```python
from build123d import *

# Parameters (mm, degrees)
SKETCH1_R            = 2.6
BASE_FLANGE1_DEPTH   = 1.524
KEYING_DEPTH         = 10
FILLET1_R            = 2
FILLET2_R            = 4
JOG1_START           = -33.370112718
JOG1_DEPTH           = 8.3
JOG1_2_DEPTH         = 8.3
JOG1_START_2         = 10.476
JOG1_3_DEPTH         = 1.524
CUT_EXTRUDE1_DEPTH   = 12
CUT_EXTRUDE1_START   = -1.524
CUT_EXTRUDE1_2_DEPTH = 1.524
CUT_EXTRUDE1_3_DEPTH = 1.524


with BuildPart() as part:
    # Base-Flange1: sheet metal written as solids
    # Sketch1 → Base-Flange1 (new body)
    with BuildSketch(Plane(origin=(0, 0, 0), x_dir=(0, 0, -1), z_dir=(1, 0, 0))):
        with BuildLine():
            Line((33.370112718, 22.8), (33.370112718, 64.8))
            Line((33.370112718, 64.8), (25.070112718, 64.8))
            Line((25.070112718, 64.8), (25.070112718, 21.281826676))
            Line((25.070112718, 21.281826676), (3.832112718, 9.020061659))
            Line((3.832112718, 9.020061659), (8.220112718, 1.419822715))
            Line((8.220112718, 1.419822715), (8.982112718, 0.1))
            Line((8.982112718, 0.1), (25.905336052, 9.870627547))
            ThreePointArc((25.905336052, 9.870627547), (31.369931839, 15.335223334), (33.370112718, 22.8))
        make_face()
        with Locations((29.220112718, 26.8)):
            Circle(SKETCH1_R, mode=Mode.SUBTRACT)
        with BuildLine():
            Line((31.720112718, 60.8), (31.720112718, 53.8))
            ThreePointArc((31.720112718, 53.8), (29.220112718, 51.3), (26.720112718, 53.8))
            Line((26.720112718, 53.8), (26.720112718, 60.8))
            ThreePointArc((26.720112718, 60.8), (29.220112718, 63.3), (31.720112718, 60.8))
        make_face(mode=Mode.SUBTRACT)
    extrude(amount=-BASE_FLANGE1_DEPTH)

    # Sketch6 → Keying (cut)
    with BuildSketch(Plane(origin=(0, 0, 0), x_dir=(0, 0, -1), z_dir=(1, 0, 0))):
        Polygon((19.287815023, 6.05), (17.763815023, 8.689645431), (13.953303246, 6.489645431), (10.14279147, 4.289645431), (11.66679147, 1.65), (15.701110868, 3.97921539), align=None)
    extrude(amount=-KEYING_DEPTH, mode=Mode.SUBTRACT)

    # Fillet1
    fillet1_edges = [part.edges().sort_by_distance(p)[0] for p in [
        (-0.762, 0.1, -8.982112718),
        (-0.762, 21.281826676, -25.070112718),
        (-0.762, 64.8, -25.070112718),
        (-0.762, 64.8, -33.370112718),
    ]]
    fillet(fillet1_edges, radius=FILLET1_R)

    # Fillet2
    fillet2_edges = [part.edges().sort_by_distance(p)[0] for p in [
        (-0.762, 9.020061659, -3.832112718),
    ]]
    fillet(fillet2_edges, radius=FILLET2_R)

    # Jog1: read off the stored shape, not the designer's step
    # Jog1 outline → Jog1 (cut)
    with BuildSketch(Plane.XY.offset(JOG1_START)):
        with BuildLine():
            ThreePointArc((-1.524, 33.004579798), (-1.115645431, 34.528579798), (0, 35.644225229))
            Line((0, 35.644225229), (0, 64.8))
            Line((0, 64.8), (-1.524, 64.8))
            Line((-1.524, 64.8), (-1.524, 33.004579798))
        make_face()
    extrude(amount=JOG1_DEPTH, mode=Mode.SUBTRACT)

    # Jog1 2 outline → Jog1 2 (add)
    with BuildSketch(Plane.XY.offset(JOG1_START)):
        with BuildLine():
            ThreePointArc((0, 33.004579798), (0.446369265, 34.082210533), (1.524, 34.528579798))
            Line((1.524, 34.528579798), (8.952, 34.528579798))
            ThreePointArc((8.952, 34.528579798), (11.107261469, 35.421318329), (12, 37.576579798))
            Line((12, 37.576579798), (12, 64.8))
            Line((12, 64.8), (10.476, 64.8))
            Line((10.476, 64.8), (10.476, 37.576579798))
            ThreePointArc((10.476, 37.576579798), (10.029630734, 36.498949063), (8.952, 36.052579798))
            Line((8.952, 36.052579798), (1.524, 36.052579798))
            ThreePointArc((1.524, 36.052579798), (0.73511955, 35.948721717), (0, 35.644225229))
            Line((0, 35.644225229), (0, 33.004579798))
        make_face()
    extrude(amount=JOG1_2_DEPTH)

    # Jog1 3 outline → Jog1 3 (cut)
    with BuildSketch(Plane.YZ.offset(JOG1_START_2)):
        with BuildLine():
            ThreePointArc((62.8, -25.070112718), (64.214213562, -25.655899156), (64.8, -27.070112718))
            Line((64.8, -27.070112718), (64.8, -25.070112718))
            Line((64.8, -25.070112718), (62.8, -25.070112718))
        make_face()
        with BuildLine():
            ThreePointArc((64.8, -31.370112718), (64.214213562, -32.78432628), (62.8, -33.370112718))
            Line((62.8, -33.370112718), (64.8, -33.370112718))
            Line((64.8, -33.370112718), (64.8, -31.370112718))
        make_face()
        with BuildLine():
            Line((60.8, -26.720112718), (53.8, -26.720112718))
            ThreePointArc((53.8, -26.720112718), (51.3, -29.220112718), (53.8, -31.720112718))
            Line((53.8, -31.720112718), (60.8, -31.720112718))
            ThreePointArc((60.8, -31.720112718), (63.3, -29.220112718), (60.8, -26.720112718))
        make_face()
    extrude(amount=JOG1_3_DEPTH, mode=Mode.SUBTRACT)

    # Cut-Extrude1: read off the stored shape, not the designer's step
    # Cut-Extrude1 outline → Cut-Extrude1 (cut)
    with BuildSketch(Plane(origin=(0, 0, 0), x_dir=(0, 0, -1), z_dir=(1, 0, 0))):
        with BuildLine():
            Line((25.070112718, 32), (33.370112718, 32))
            Line((33.370112718, 32), (33.370112718, 62.8))
            ThreePointArc((33.370112718, 62.8), (32.78432628, 64.214213562), (31.370112718, 64.8))
            Line((31.370112718, 64.8), (27.070112718, 64.8))
            ThreePointArc((27.070112718, 64.8), (25.655899156, 64.214213562), (25.070112718, 62.8))
            Line((25.070112718, 62.8), (25.070112718, 32))
        make_face()
        with BuildLine():
            ThreePointArc((26.720112718, 60.8), (29.220112718, 63.3), (31.720112718, 60.8))
            Line((31.720112718, 60.8), (31.720112718, 53.8))
            ThreePointArc((31.720112718, 53.8), (29.220112718, 51.3), (26.720112718, 53.8))
            Line((26.720112718, 53.8), (26.720112718, 60.8))
        make_face(mode=Mode.SUBTRACT)
    extrude(amount=CUT_EXTRUDE1_DEPTH, mode=Mode.SUBTRACT)

    # Cut-Extrude1 2 outline → Cut-Extrude1 2 (cut)
    with BuildSketch(Plane(origin=(0, 0, 0), x_dir=(0, 0, -1), z_dir=(1, 0, 0)).offset(CUT_EXTRUDE1_START)):
        with BuildLine():
            ThreePointArc((28.220112718, 35.3), (27.720112718, 34.8), (28.220112718, 34.3))
            Line((28.220112718, 34.3), (30.220112718, 34.3))
            ThreePointArc((30.220112718, 34.3), (30.720112718, 34.8), (30.220112718, 35.3))
            Line((30.220112718, 35.3), (28.220112718, 35.3))
        make_face()
    extrude(amount=CUT_EXTRUDE1_2_DEPTH, mode=Mode.SUBTRACT)

    # Cut-Extrude1 3 outline → Cut-Extrude1 3 (add)
    with BuildSketch(Plane(origin=(0, 0, 0), x_dir=(0, 0, -1), z_dir=(1, 0, 0)).offset(CUT_EXTRUDE1_START)):
        with BuildLine():
            Line((25.070112718, 32), (33.370112718, 32))
            Line((33.370112718, 32), (33.370112718, 72.837680806))
            ThreePointArc((33.370112718, 72.837680806), (32.78432628, 74.251894368), (31.370112718, 74.837680806))
            Line((31.370112718, 74.837680806), (27.070112718, 74.837680806))
            ThreePointArc((27.070112718, 74.837680806), (25.655899156, 74.251894368), (25.070112718, 72.837680806))
            Line((25.070112718, 72.837680806), (25.070112718, 32))
        make_face()
        with BuildLine():
            ThreePointArc((28.220112718, 34.3), (27.720112718, 34.8), (28.220112718, 35.3))
            Line((28.220112718, 35.3), (30.220112718, 35.3))
            ThreePointArc((30.220112718, 35.3), (30.720112718, 34.8), (30.220112718, 34.3))
            Line((30.220112718, 34.3), (28.220112718, 34.3))
        make_face(mode=Mode.SUBTRACT)
        with BuildLine():
            Line((28.220112718, 46.318840403), (30.220112718, 46.318840403))
            ThreePointArc((30.220112718, 46.318840403), (30.720112718, 45.818840403), (30.220112718, 45.318840403))
            Line((30.220112718, 45.318840403), (28.220112718, 45.318840403))
            ThreePointArc((28.220112718, 45.318840403), (27.720112718, 45.818840403), (28.220112718, 46.318840403))
        make_face(mode=Mode.SUBTRACT)
        with BuildLine():
            Line((26.720112718, 63.837680806), (26.720112718, 70.837680806))
            ThreePointArc((26.720112718, 70.837680806), (29.220112718, 73.337680806), (31.720112718, 70.837680806))
            Line((31.720112718, 70.837680806), (31.720112718, 63.837680806))
            ThreePointArc((31.720112718, 63.837680806), (29.220112718, 61.337680806), (26.720112718, 63.837680806))
        make_face(mode=Mode.SUBTRACT)
    extrude(amount=CUT_EXTRUDE1_3_DEPTH)


solid = part.part
```
Part model, mm, in its own coordinate system. A direction names the side the tool comes from. Coordinates: 2 decimals unless noted, no trailing zeros. Write each loop counter-clockwise with the first axis right and the second up, starting at its lowest first coordinate (ties: lowest second). Pieces come first, ordered by that corner, then holes.
Item 1: Slice it at A-A (y = 26.8). Write the cut outline in (x, z).
Item 2: Slice it at C-C (z = -20.75). Write the cut outline in (x, y), and give its area (3 significant figures).
Item 3: Pin check, flat tip, straight feed: pin 1 (0.5 mm diameter, centred on x = -0.5, y = 67.5, fed in from +Z). Stop position of the tip, or through.
Item 4: Slice it at B-B (y = 48.5). Write the cut outline in (x, z).
Item 5: Mould opens along Z. For faces 1 (the face through (-0.77, 21.45, -24.81)), 2 (the face through (0, 30, -27)), 3 (the face through (-1, 46.319, -29)), 4 (the face through (-0.751, 2.988, -10.894)) say: released by +Z, released by -Z, zero draft, split by the parting line, or undercut.
Item 6: Probe line 1 (Z direction, x = -0.05, y = 69); line 2 (Y direction, x = -0.55, z = -30); line 3 (Z direction, x = -0.7, y = 47.5). List the from-to ranges inside material, lowest first.
Item 7: Which spindle directions (+Z, -Z, +X, -X, +Y, -Y) get a long thin tool onto all of the face, cutting with end or side? Do faces 5 (the face through (-1, 67, -26.72)), 6 (the face through (-0.75, 3.72, -6.89)), 7 (the face through (-1, 48, -25.07)). Say none if no direction does.
Results found:
1. outline: (-1.52, -33.37) - (0, -33.37) - (0, -31.82) - (-1.52, -31.82) - close; (-1.52, -26.62) - (0, -26.62) - (0, -25.07) - (-1.52, -25.07) - close
2. outline: (-1.52, 6.89) - (0, 6.89) - (0, 18.79) - (-1.52, 18.79) - close
2. area: 18.1 mm2
3. pin 1: stops at z = -25.07
4. outline: (-1.52, -33.37) - (0, -33.37) - (0, -25.07) - (-1.52, -25.07) - close
5. face 1: released by +Z
5. face 2: zero draft
5. face 3: undercut
5. face 4: released by -Z
6. line 1: z = -33.37 to -31.72, -26.72 to -25.07
6. line 2: y = 13.35 to 24.32, 29.28 to 34.3, 35.3 to 45.32, 46.32 to 61.46, 73.21 to 74.84
6. line 3: z = -33.37 to -25.07
7. face 5: +X, -X
7. face 6: +Z, +X, -X, -Y
7. face 7: +Z, +X, -X, +Y
